Design review of the part built by this model. Coordinates are the model's own, in mm. A direction names the side the tool comes from. Give positions to 0.01 mm unless a question says otherwise; leave off trailing zeros. Order: outer loops, then holes, each group sorted by start corner. A loop starts at its lowest first (then second) coordinate and runs counter-clockwise, first axis right, second up. Notation, with made-up numbers: (-23, 22.25) -> (36, 22.25) arc R21 ccw to (36, 47.25) -> close; hole circle Ø5 at (20, 84). An arc over 180 degrees is marked (long way). One line per item, written item: value. Start each with the question number.
1) Wall thickness on line 1 along Y through (x, z) = (0, 101); line 2 along Y through (x, z) = (-0.25, 375); line 3 along Y through (x, z) = (9.25, 277.5): over which ranges is each line inside the solid? List them lowest first. Write a range as from..to.
2) Consider section B-B (z = 317). State the section outline as (x, y) points, plus the area to 3 significant figures.
3) For pin 1 (9.5 mm diameter, centred on x = -2.5, y = 0.5, fed in from -Z); pin 2 (12 mm diameter, centred on x = 5.5, y = 7, fed in from +Z); pin 3 (5 mm diameter, centred on y = -6.5, z = 126, fed in from -X); pin 4 (1 mm diameter, centred on y = 6, z = 392.5, fed in from +X), all flat-tipped, find the tip position at first contact; note any pin that passes through.
4) Tool access review of faces 1 (the face through (6, 0, 100)), 2 (the face through (-3.687, 0.084, 464.144)): name each direction out of +Z, -Z, +X, -X, +Y, -Y from which nothing blocks a thin tool from reaching the whole face with its end or side.
5) Consider section A-A (y = 0). State the section outline as (x, z) points.
6) The part is to be moulded in two halves that separate along X. For faces 3 (the face through (-2.17, -9.76, 288.58)), 4 (the face through (0, 0, 118)), 5 (the face through (7, 0, 83)), 6 (the face through (0.14, 6.527, 498.934)), say which applies: released by +X, released by -X, zero draft, split by the parting line, or undercut.
from build123d import *

# Parameters (mm, degrees)
SZKIC1_R                        = 10
DODANIE_WYCI_GNI_CIE1_DEPTH     = 500
SZKIC2_R                        = 6
WYTNIJ_WYCI_GNI_CIE1_DEPTH      = 118
WYTNIJ_WYCI_GNI_CIE2_DEPTH      = 35
WYTNIJ_WYCI_GNI_CIE2_DEPTH_BACK = 35
SZKIC4_R                        = 6
WYTNIJ_WYCI_GNI_CIE3_DEPTH      = 35
WYTNIJ_WYCI_GNI_CIE4_DEPTH      = 20
WYTNIJ_WYCI_GNI_CIE4_DEPTH_BACK = 20
SZKIC5_W                        = 20
SZKIC5_H                        = 83


with BuildPart() as part:
    # Szkic1 → Dodanie-wyciągnięcie1 (new body)
    with BuildSketch(Plane.XY):
        Circle(SZKIC1_R)
    extrude(amount=DODANIE_WYCI_GNI_CIE1_DEPTH)

    # Szkic2 → Wytnij-wyciągnięcie1 (cut)
    with BuildSketch(Plane(origin=(0, 0, 0), x_dir=(-1, 0, 0), z_dir=(0, 0, -1))):
        Circle(SZKIC2_R)
    extrude(amount=-WYTNIJ_WYCI_GNI_CIE1_DEPTH, mode=Mode.SUBTRACT)

    # Szkic3 → Wytnij-wyciągnięcie2 (cut, two sides: drawn at the far end of the back side and taken through both)
    with BuildSketch(Plane(origin=(0, 0, 0), x_dir=(1, 0, 0), z_dir=(0, 1, 0)).offset(-WYTNIJ_WYCI_GNI_CIE2_DEPTH_BACK)):
        Polygon((-10, -500), (10, -500), (15.054630998, -497.366652169), align=None)
    extrude(amount=WYTNIJ_WYCI_GNI_CIE2_DEPTH + WYTNIJ_WYCI_GNI_CIE2_DEPTH_BACK, mode=Mode.SUBTRACT)

    # Szkic4 → Wytnij-wyciągnięcie3 (cut)
    with BuildSketch(Plane(origin=(51.868660708, 0, 493.497341729), x_dir=(0.9945218953682733, 0, -0.10452846326765462), z_dir=(0.10452846326765461, 0, 0.9945218953682732))):
        with Locations((-52.099435871, 0)):
            Circle(SZKIC4_R)
    extrude(amount=-WYTNIJ_WYCI_GNI_CIE3_DEPTH, mode=Mode.SUBTRACT)

    # Szkic5 → Wytnij-wyciągnięcie4 (cut, two sides: drawn at the far end of the back side and taken through both)
    with BuildSketch(Plane(origin=(0, 0, 0), x_dir=(1, 0, 0), z_dir=(0, 1, 0)).offset(-WYTNIJ_WYCI_GNI_CIE4_DEPTH_BACK)):
        with Locations((0, -41.5)):
            Rectangle(SZKIC5_W, SZKIC5_H)
    extrude(amount=WYTNIJ_WYCI_GNI_CIE4_DEPTH + WYTNIJ_WYCI_GNI_CIE4_DEPTH_BACK, mode=Mode.SUBTRACT)


solid = part.part
Checked values:
1. line 1: y = -10..-6, 6..10
1. line 2: y = -10..10
1. line 3: y = -3.8..3.8
2. outline: circle Ø20 at (0, 0)
2. area: 314 mm^2
3. pin 1: stops at z = 83
3. pin 2: stops at z = 499
3. pin 3: stops at x = -9.17
3. pin 4: stops at x = 8.35
4. face 1: -Z
4. face 2: none
5. outline: (-10, 83) -> (-6, 83) -> (-6, 118) -> (6, 118) -> (6, 83) -> (10, 83) -> (10, 497.9) -> (6.02, 498.32) -> (2.36, 463.51) -> (-9.57, 464.76) -> (-5.91, 499.57) -> (-10, 500) -> close
6. face 3: split by the parting line
6. face 4: undercut
6. face 5: zero draft
6. face 6: released by +X
